The drawing under review shows one solid part. Ordinate dimensions are in mm from its lowest x, y, z. A direction names the side the tool comes from. Coordinates: 2 decimals unless noted, no trailing zeros. Order: outer loops, then holes, each group sorted by start corner. A loop starts at its lowest first (then second) coordinate and runs counter-clockwise, first axis right, second up.
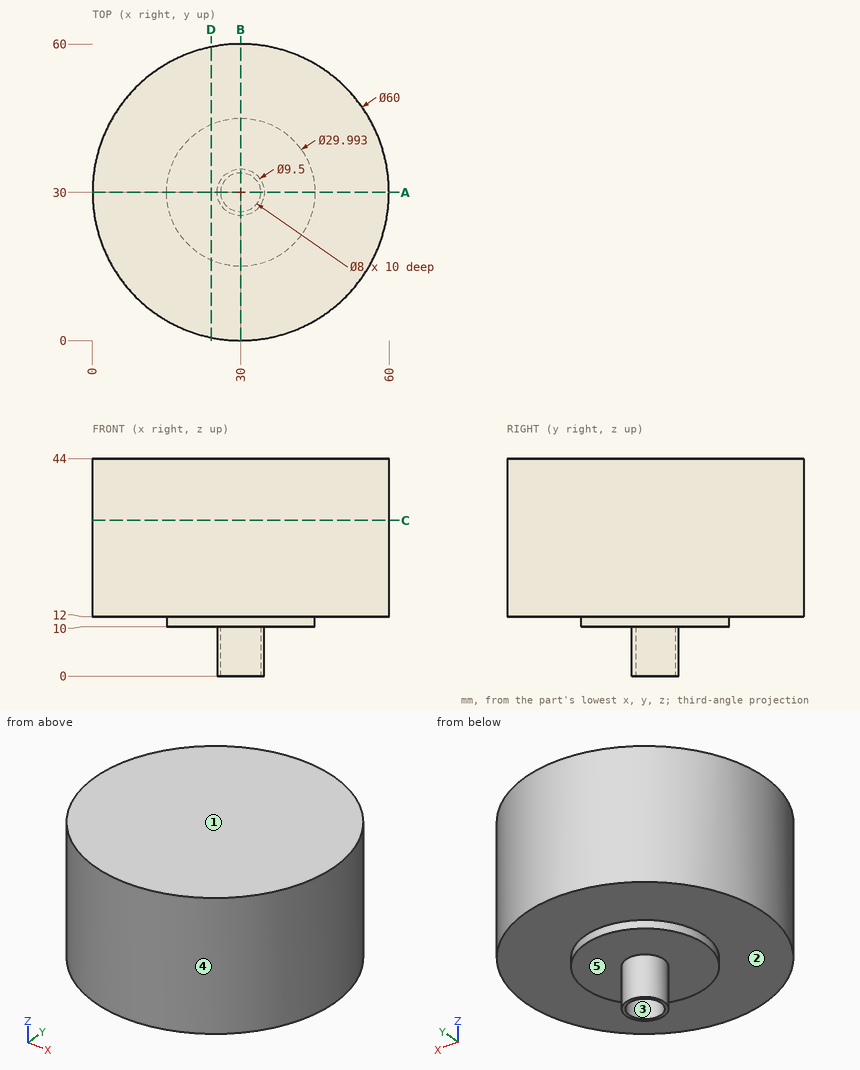
1. Insertion check: pin 1 (1 mm diameter, centred on y = 35, z = 27, fed in from +X); pin 2 (12 mm diameter, centred on x = 45.5, y = 48.5, fed in from -Z); pin 3 (3 mm diameter, centred on x = 18, z = 29.5, fed in from +Y). Each pin has a flat end and moves straight along its axis. Give the tip position at first contact, or say it passes through.
2. For the marked faces 1 and 2, list the 3-axis set-ups (+Z, -Z, +X, -X, +Y, -Y) from which the entire face can be reached by the end or side of a thin tool; tool diameter is ignored.
3. Mouldability with a two-part tool opening along X and no side actions: class the marked faces 3, 4 and 5 as pulls with the +X half, pulls with the -X half, needs draft (parallel to the pull), parting line crosses it, or undercut.
4. Add section A-A (y = 30). Give the boundary of the cut face in (x, z), and give its area (4 significant figures).
5. Add section C-C (z = 31.5). Give the boundary of the cut face in (x, y).
6. Add section D-D (x = 24). Give the boundary of the cut face in (y, z), and give its area (3 significant figures).
7. To check wall thickness, follow line 1 (Y direction, x = 30, z = 5.25); line 2 (Z direction, x = 20, y = 25); line 3 (Z direction, x = 50.5, y = 19.5). State the ranges of each line that lie inside material, in increasing order.
Solution:
1. pin 1: stops at x = 59.66
1. pin 2: stops at z = 12
1. pin 3: stops at y = 58.1
2. face 1: +Z, +X, -X, +Y, -Y
2. face 2: -Z
3. face 3: undercut
3. face 4: parting line crosses it
3. face 5: needs draft
4. outline: (0, 12) - (15, 12) - (15, 10) - (25.25, 10) - (25.25, 0) - (26, 0) - (26, 10) - (34, 10) - (34, 0) - (34.75, 0) - (34.75, 10) - (45, 10) - (45, 12) - (60, 12) - (60, 44) - (0, 44) - close
4. area: 1,995 mm2
5. outline: circle Ø60 at (30, 30)
6. outline: (0.61, 12) - (16.26, 12) - (16.26, 10) - (43.74, 10) - (43.74, 12) - (59.39, 12) - (59.39, 44) - (0.61, 44) - close
6. area: 1,940 mm2
7. line 1: y = 25.25 to 26, 34 to 34.75
7. line 2: z = 10 to 44
7. line 3: z = 12 to 44
